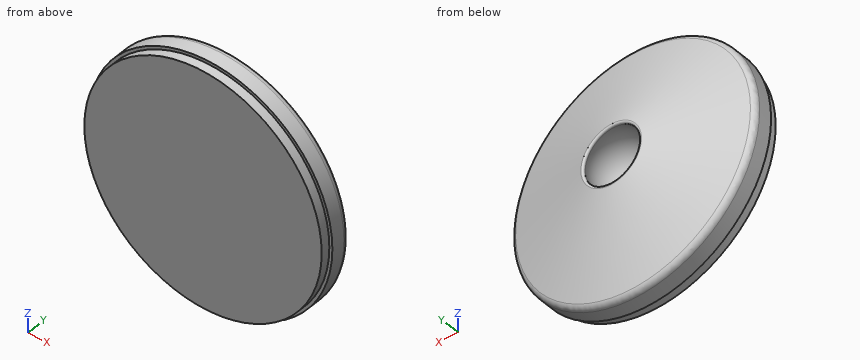
from build123d import *

# Parameters (mm, degrees)
FILLET1_R           = 0.3
SKETCH4_R           = 19.5
BOSS_EXTRUDE1_DEPTH = 1.5
FILLET2_R           = 1


with BuildPart() as part:
    # Sketch2 → Revolve1 (revolve)
    with BuildSketch(Plane.XY):
        Polygon((0, 0), (-20, 0), (-20, 3.004926108), (0, 9.014778325), align=None)
    revolve(axis=Axis((0, 35.024630542, 0), (0, -1, 0)))

    # Sketch3 → Cut-Revolve2 (revolve, cut)
    with BuildSketch(Plane.XY):
        with BuildLine():
            Line((0, 0.2), (0, 10.2))
            ThreePointArc((0, 10.2), (-5, 5.2), (0, 0.2))
        make_face()
    revolve(axis=Axis((0, 12.296737064, 0), (0, -1, 0)), mode=Mode.SUBTRACT)

    # Fillet1
    fillet1_edges = [part.edges().sort_by_distance(p)[0] for p in [
        (4.320571191, 7.716478608, 0),
    ]]
    fillet(fillet1_edges, radius=FILLET1_R)

    # Sketch4 → Boss-Extrude1 (add)
    with BuildSketch(Plane.XZ):
        Circle(SKETCH4_R)
    extrude(amount=BOSS_EXTRUDE1_DEPTH)

    # Fillet2
    fillet2_edges = [part.edges().sort_by_distance(p)[0] for p in [
        (20, 3.004926108, 0),
    ]]
    fillet(fillet2_edges, radius=FILLET2_R)


solid = part.part
Work out the finished part from the listing and answer in its coordinate system (mm). Round coordinates to 2 decimals unless told otherwise and drop trailing zeros. Loops run counter-clockwise (first coordinate to the right, second up) from the corner with the lowest first, then second, coordinate; pieces in that order, holes last. Notation, with made-up numbers: (38.25, 40) - (65.25, 40) arc R28 ccw to (65.25, 65) - close; hole circle Ø10 at (-15.5, 25). An arc over 180 degrees is marked (long way). One line per item, written item: value.
Q1. Each of these flat-tipped pins is pushed along its axis until it touches: pin 1 Ø5 at (x, z) = (-13, 5.5) entering from +Y; pin 2 Ø1 at (x, y) = (9.5, 3) entering from +Z; pin 3 Ø4 at (y, z) = (1, -8.5) entering from +X. Where does it stop, or does it pass through?
Check values:
pin 1: y = 5.52
pin 2: z = 17.7
pin 3: x = 18.91
Q2. Find section A-A on y = -0.5. Give the vertices of the cut face in (x, z), and give its area (3 significant figures).
Check values:
outline: circle Ø39 at (0, 0)
area: 1,190 mm2
Q3. Find section B-B on y = 6. Give the vertices of the cut face in (x, z), and give its area (3 significant figures).
Check values:
outline: circle Ø20.07 at (0, 0); hole circle Ø9.87 at (0, 0)
area: 240 mm2
Q4. Straight lines are drawn through the part: probe 1 along X at (y, z) = (1, 1); probe 2 along X at (y, z) = (2.5, 1); probe 3 along Y at (x, z) = (3.5, -17.5). For each, find the intervals that lie inside material, in ascending order.
Check values:
probe 1: -19.97 to -2.52, 2.52 to 19.97
probe 2: -19.95 to -4.09, 4.09 to 19.95
probe 3: -1.5 to 3.65
